Autodesk Inventor part; units mm, degrees
ref_plane "YZ Plane" through (0, 0, 0) normal (1, 0, 0) x (0, 1, 0)
ref_plane "XZ Plane" through (0, 0, 0) normal (0, 1, 0) x (-1, 0, 0)
ref_plane "XY Plane" through (0, 0, 0) normal (0, 0, 1) x (1, 0, 0)
sketch "Sketch1" plane through (0, 0, 0) normal (0, 1, 0) x (-1, 0, 0)
  arc A0 (7.808, 86.5621) -> (-1.4957, 90.4158) centre (2.358, 86.5621) ccw
  line L0 (7.808, 86.5621) -> (7.808, -83.4379)
  line L1 (-1.4957, 90.4158) -> (-12.3494, 79.5621)
  arc A1 (-12.3494, 79.5621) -> (-14.4205, 74.5621) centre (-7.3494, 74.5621) ccw
  line L2 (-14.4205, 74.5621) -> (-14.4205, -71.4379)
  arc A2 (-1.4957, -87.2917) -> (7.808, -83.4379) centre (2.358, -83.4379) ccw
  line L3 (-1.4957, -87.2917) -> (-12.3494, -76.4379)
  arc A3 (-14.4205, -71.4379) -> (-12.3494, -76.4379) centre (-7.3494, -71.4379) ccw
  point P0 (0, 0)
  dimension "d0" = 10.9
  dimension "d1" = 170
  dimension "d2" = 0
  dimension "d3" = 12
  dimension "d4" = 12
  dimension "d5" = 5.45
  dimension "d6" = 45
  dimension "d7" = 7
  dimension "d8" = 7
  dimension "d9" = 10.9
  dimension "d10" = 135
extrude "Extrusion1" add sketch "Sketch1" along normal blind 1.7
sketch "Sketch2" plane through (0, 1.7, 0) normal (0, 1, 0) x (1, 0, 0)
  arc A0 (1.4957, 87.2917) -> (-7.808, 83.4379) centre (-2.358, 83.4379) ccw
  arc A1 (-7.808, -86.5621) -> (1.4957, -90.4158) centre (-2.358, -86.5621) ccw
  circle A2 centre (-2.358, 83.4379) radius 3
  circle A3 centre (-2.358, -86.5621) radius 1.5
  point P0 (0, 0)
  dimension "d13" = 6
  dimension "d14" = 3
extrude "Extrusion2" cut sketch "Sketch2" against normal through all
properties part number "A2P4"
CAD build for the part. Positions are in the model's coordinates, mm. Coordinates: 2 decimals unless noted, no trailing zeros. Loops run counter-clockwise (first coordinate to the right, second up) from the corner with the lowest first, then second, coordinate; pieces in that order, holes last. Notation, with made-up numbers: (77.25, -39) - (84.25, -39) arc R25 ccw to (84.25, -19) - close; hole circle Ø10 at (-21.75, 2). An arc over 180 degrees is marked (long way). Use one line per item in the form item = value. Start each with the question number.
1) Band-saw the part on B-B (x = 6.5). Give the cut face in (y, z).
2) Two-plate mould, pull along X, no slides. Class faces 1 (the face through (3, 0, 3)), 2 (the face through (-2.749, 0.862, -86.412)), 3 (the face through (6.85, 0.84, -81.94)), 4 (the face through (-1.666, 0.862, 87.893)): +X half, -X half, draft (parallel to the pull), parting line (faces both ways), or undercut.
3) Drill centre lines: L1, parallel to Z at x = -2.5, y = 0.35; L2, parallel to Z at x = 1.5, y = 0.1; L3, parallel to Z at x = -0.5, y = 1.6. Where is each one in solid material? Low to high. Write a range as from..to.
4) Band-saw the part on A-A (y = 1.3). Give the cut face in (x, z), and give its area (3 significant figures).
Check values:
q1.outline = (0, -82.29) - (1.7, -82.29) - (1.7, 85.41) - (0, 85.41) - close
q2.face_1 = draft
q2.face_2 = undercut
q2.face_3 = +X half
q2.face_4 = undercut
q3.L1 = -88.89..-86.43, -80.44..85.07, 88.06..92.01
q3.L2 = -87.29..90.41
q3.L3 = -88.56..-85.79, -81.08..91.69
q4.outline = (-7.81, -83.44) arc R5.45 ccw to (1.5, -87.29) - (12.35, -76.44) arc R7.07 ccw to (14.42, -71.44) - (14.42, 74.56) arc R7.07 ccw to (12.35, 79.56) - (1.5, 90.42) arc R5.45 ccw to (-7.81, 86.56) - close; hole circle Ø6 at (-2.36, -83.44); hole circle Ø3 at (-2.36, 86.56)
q4.area = 3,760 mm2
